Part model, mm, in its own coordinate system. A direction names the side the tool comes from. Round coordinates to 2 decimals unless told otherwise and drop trailing zeros. Write each loop counter-clockwise with the first axis right and the second up, starting at its lowest first coordinate (ties: lowest second). Pieces come first, ordered by that corner, then holes. Notation, with made-up numbers: M 41.5,32.25 L 55.5,32.25 A22 cw 55.5,40.25 Z; hole C 59,65.5 d9. An arc over 180 degrees is marked long. Use one line per item in the form item = value. Start each with the question number.
Item 1: Cut at D-D, the plane y = -0.5. Give the cut face in (x, z), then the cut area to 3 significant figures.
Item 2: Which spindle directions (+Z, -Z, +X, -X, +Y, -Y) get a long thin tool onto all of the face, cutting with end or side? Do faces 1 (the face through (12, 0, 7.112)), 2 (the face through (-20.593, 7.022, 11.214)), 3 (the face through (20.6, 6.5, 11.4)). Say none if no direction does.
Item 3: Cut at B-B, the plane z = 10.16. Give the cut face in (x, y).
Item 4: Probe L1, parallel to X at y = 1.5, z = 10.5; L2, parallel to Z at x = 21.5, y = -6.35; L3, parallel to Z at x = 8, y = -2.25. List the from-to ranges inside material, lowest first.
Item 5: Cut at C-C, the plane x = 20.5. Give the cut face in (y, z), then the cut area to 3 significant figures.
Item 6: Flat gauge pins, fed straight in: pin 1 Ø2 at (y, z) = (6.35, 10.16) entering from +X; pin 2 Ø3.5 at (x, y) = (-13.5, -6) entering from +Z. Where does each tip first touch, or does it go through?
Item 7: Cut at A-A, the plane y = -6.35. Give the cut face in (x, z), then the cut area to 3 significant figures.
Item 8: Mould opens along X. For faces 4 (the face through (-17.462, 0, 10)), 5 (the face through (0, 0, 12.7)), 6 (the face through (-5.728, 0, 10)), 7 (the face through (23.812, 0, 6)) say: +X half, -X half, draft (parallel to the pull), parting line (faces both ways), or undercut.
from build123d import *

# Parameters (mm, degrees)
F0_W     = 47.625
F0_H     = 25.4
F1_DEPTH = 12.7
F2_W     = 11.7348
F2_H     = 25.4
F3_DEPTH = 5.588
F6_D     = 2.5
F6_DEPTH = 7.62
F6_TIP   = 0.7510757738
F7_D     = 2.5
F7_DEPTH = 7.62
F7_TIP   = 0.7510757738


with BuildPart() as f1:
    # F0 (on Top) → F1 (new body)
    with BuildSketch(Plane.XY):
        Rectangle(F0_W, F0_H)
    extrude(amount=F1_DEPTH)

    # F2 (on face) → F3 (cut)
    with BuildSketch(Plane.XY.offset(12.7)):
        with Locations((-11.5951, 0)):
            Rectangle(F2_W, F2_H)
        with Locations((11.5951, 0)):
            Rectangle(F2_W, F2_H)
    extrude(amount=-F3_DEPTH, mode=Mode.SUBTRACT)

    # F6
    with Locations(Plane(origin=(-23.8125, 0, 0), x_dir=(0, -1, 0), z_dir=(-1, 0, 0))):
        with Locations((6.35, 10.16), (-6.35, 10.16)):
            Hole(F6_D / 2, depth=F6_DEPTH)
            with Locations((0, 0, -(F6_DEPTH + F6_TIP / 2))):  # 118° drill point
                Cone(0, F6_D / 2, F6_TIP, mode=Mode.SUBTRACT)

    # F7
    with Locations(Plane.YZ.offset(23.8125)):
        with Locations((-6.35, 10.16), (6.35, 10.16)):
            Hole(F7_D / 2, depth=F7_DEPTH)
            with Locations((0, 0, -(F7_DEPTH + F7_TIP / 2))):  # 118° drill point
                Cone(0, F7_D / 2, F7_TIP, mode=Mode.SUBTRACT)


solid = f1.part
Model answer:
q1.outline = M -23.81,0 L 23.81,0 L 23.81,12.7 L 17.46,12.7 L 17.46,7.11 L 5.73,7.11 L 5.73,12.7 L -5.73,12.7 L -5.73,7.11 L -17.46,7.11 L -17.46,12.7 L -23.81,12.7 Z
q1.area = 474 mm²
q2.face_1 = +Z, +Y, -Y
q2.face_2 = -X
q2.face_3 = +X
q3.outline = M -23.81,-12.7 L -17.46,-12.7 L -17.46,-7.6 L -23.81,-7.6 Z; M -23.81,-5.1 L -17.46,-5.1 L -17.46,5.1 L -23.81,5.1 Z; M -23.81,7.6 L -17.46,7.6 L -17.46,12.7 L -23.81,12.7 Z; M -5.73,-12.7 L 5.73,-12.7 L 5.73,12.7 L -5.73,12.7 Z; M 17.46,-12.7 L 23.81,-12.7 L 23.81,-7.6 L 17.46,-7.6 Z; M 17.46,-5.1 L 23.81,-5.1 L 23.81,5.1 L 17.46,5.1 Z; M 17.46,7.6 L 23.81,7.6 L 23.81,12.7 L 17.46,12.7 Z
q4.L1 = -23.81 to -17.46, -5.73 to 5.73, 17.46 to 23.81
q4.L2 = 0 to 8.91, 11.41 to 12.7
q4.L3 = 0 to 7.11
q5.outline = M -12.7,0 L 12.7,0 L 12.7,12.7 L -12.7,12.7 Z; hole C -6.35,10.16 d2.5; hole C 6.35,10.16 d2.5
q5.area = 313 mm²
q6.pin_1 = 5.73
q6.pin_2 = 7.11
q7.outline = M -23.81,0 L 23.81,0 L 23.81,8.91 L 17.46,8.91 L 17.46,7.11 L 5.73,7.11 L 5.73,12.7 L -5.73,12.7 L -5.73,7.11 L -17.46,7.11 L -17.46,8.91 L -23.81,8.91 Z; M -23.81,11.41 L -17.46,11.41 L -17.46,12.7 L -23.81,12.7 Z; M 17.46,11.41 L 23.81,11.41 L 23.81,12.7 L 17.46,12.7 Z
q7.area = 442 mm²
q8.face_4 = undercut
q8.face_5 = draft
q8.face_6 = undercut
q8.face_7 = +X half
